Part print with two shaded views. Sizes in mm from the minimum x, y, z corner. A direction names the side the tool comes from. Round coordinates to 2 decimals unless told otherwise and drop trailing zeros. Loops run counter-clockwise (first coordinate to the right, second up) from the corner with the lowest first, then second, coordinate; pieces in that order, holes last. Notation, with made-up numbers: M -11.75,40 L -0.75,40 A29 ccw -0.75,73 Z; hole C 33,51.5 d9. An arc over 180 degrees is marked long. Answer as CSV lines item,"result". Start each with the question number.
Item 1: Band-saw the part on A-A (y = 2.5). Give the cut face in (x, z), and give its area (3 significant figures).
Item 2: Which spindle directions (+Z, -Z, +X, -X, +Y, -Y) get a long thin tool onto all of the face, cutting with end or side? Do the marked faces 1, 2 and 3. Say none if no direction does.
Item 3: Band-saw the part on C-C (x = 18.75). Give the cut face in (y, z), and give its area (3 significant figures).
Item 4: Band-saw the part on B-B (x = 5). Give the cut face in (y, z).
Item 5: Drop flat-ended pins along their axis: pin 1 Ø3.5 at (x, y) = (5, 2.5) entering from +Z; pin 2 Ø8 at (x, y) = (14.5, 49) entering from +Z; pin 3 Ø5.5 at (x, y) = (15, 2.5) entering from -Z; pin 4 Ø5 at (x, z) = (10, 35) entering from +Y. Give the stop position or say it passes through.
Item 6: Wall check: line 1 (X direction, y = 52, z = 29); line 2 (Y direction, x = 15, z = 30.2); line 3 (X direction, y = 2, z = 29). Give the ranges that are in metal, low to high.
Item 7: Band-saw the part on D-D (z = 7.5). Give the cut face in (x, y).
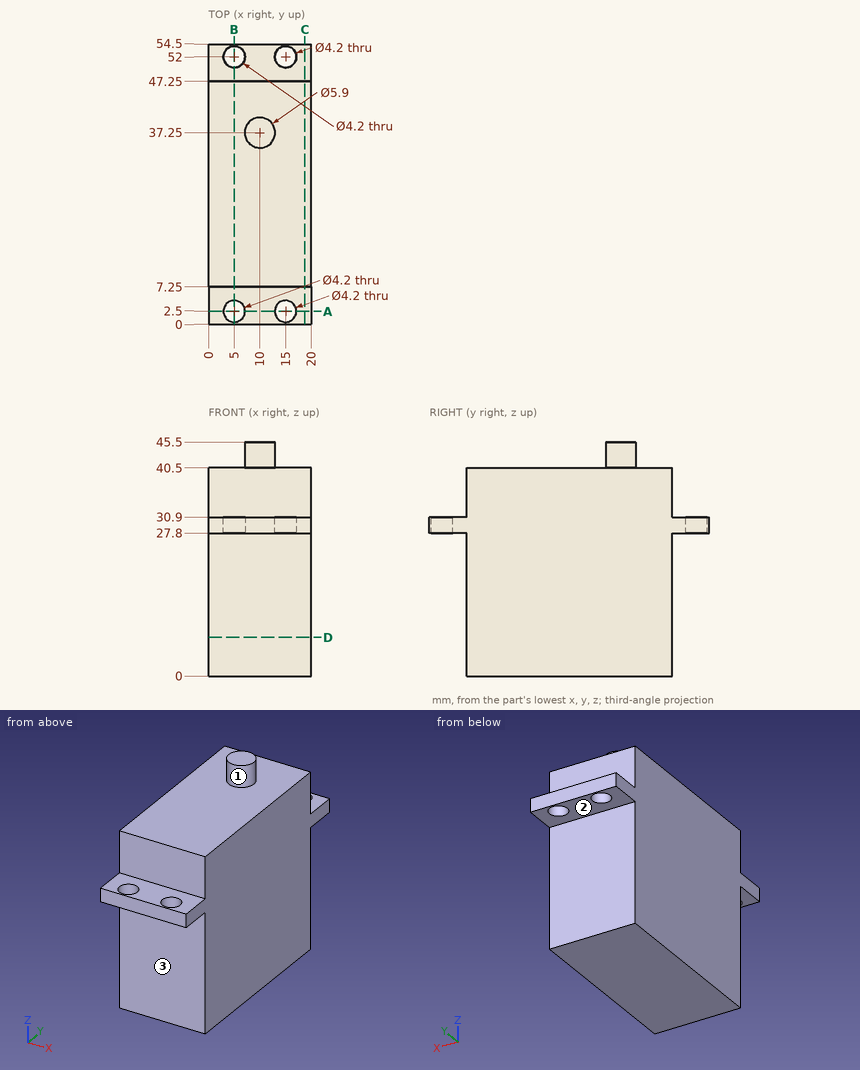
Answer block:
1,outline,"M 0,27.8 L 2.9,27.8 L 2.9,30.9 L 0,30.9 Z; M 7.1,27.8 L 12.9,27.8 L 12.9,30.9 L 7.1,30.9 Z; M 17.1,27.8 L 20,27.8 L 20,30.9 L 17.1,30.9 Z"
1,area,"36.0 mm^2"
2,face 1,"+Z"
2,face 2,"-Z, +X, -X, +Y"
2,face 3,"-Z, +X, -X, -Y"
3,outline,"M 0,27.8 L 7.25,27.8 L 7.25,0 L 47.25,0 L 47.25,27.8 L 54.5,27.8 L 54.5,30.9 L 47.25,30.9 L 47.25,40.5 L 7.25,40.5 L 7.25,30.9 L 0,30.9 Z"
3,area,"1,660 mm^2"
4,outline,"M 0,27.8 L 0.4,27.8 L 0.4,30.9 L 0,30.9 Z; M 4.6,27.8 L 7.25,27.8 L 7.25,0 L 47.25,0 L 47.25,27.8 L 49.9,27.8 L 49.9,30.9 L 47.25,30.9 L 47.25,40.5 L 7.25,40.5 L 7.25,30.9 L 4.6,30.9 Z; M 54.1,27.8 L 54.5,27.8 L 54.5,30.9 L 54.1,30.9 Z"
5,pin 1,"passes through"
5,pin 2,"stops at z = 40.5"
5,pin 3,"stops at z = 27.8"
5,pin 4,"stops at y = 47.25"
6,line 1,"x = 0 to 2.9, 7.1 to 12.9, 17.1 to 20"
6,line 2,"y = 0 to 0.4, 4.6 to 49.9, 54.1 to 54.5"
6,line 3,"x = 0 to 2.96, 7.04 to 12.96, 17.04 to 20"
7,outline,"M 0,7.25 L 20,7.25 L 20,47.25 L 0,47.25 Z"
